Source: three-view drawing plus pictorial views. Frame: mm from the lowest corner of the part. Round coordinates to 2 decimals unless told otherwise and drop trailing zeros. Loops run counter-clockwise (first coordinate to the right, second up) from the corner with the lowest first, then second, coordinate; pieces in that order, holes last. Notation, with made-up numbers: M -16.75,47 L 8.25,47 A22 ccw 8.25,81 Z; hole C 5.25,-24 d4. An arc over 180 degrees is marked long. Write each question's results on one line, items separated by ' | '.
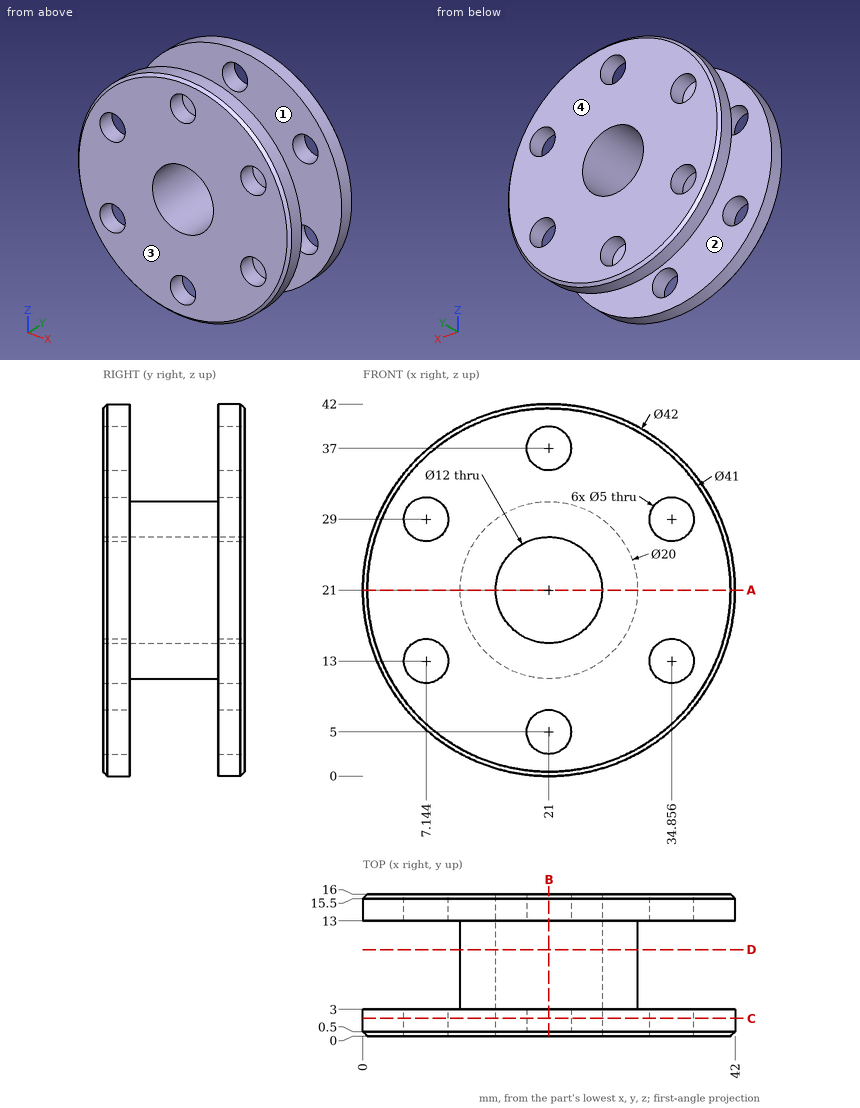
1. Pin query (flat end, axial travel): P1, Ø3, axis at x = 7.14, z = 13, coming from the -Y side; P2, Ø6, axis at x = 25.5, y = 11.5, coming from the +Z side; P3, Ø2, axis at x = 17, y = 7, coming from the +Z side; P4, Ø4, axis at x = 26, y = 12.5, coming from the -Z side (1 decimal). Return the tip coordinate at first contact, or that it passes through.
Answer key:
P1: passes through | P2: stops at z = 41.91 | P3: stops at z = 30.54 | P4: stops at z = 0.2
2. Ray query, probe 1 along Z at (x, y) = (21, 15.1); probe 2 along Z at (x, y) = (22, 15) (1 decimal); probe 3 along Y at (x, z) = (32, 18). Return the intervals inside material, ascending.
Answer key:
probe 1: z = 0 to 2.5, 7.5 to 15, 27 to 34.5, 39.5 to 42 | probe 2: z = 0 to 2.7, 7.3 to 15.1, 26.9 to 34.7, 39.3 to 42 | probe 3: y = 0 to 3, 13 to 16
3. Section D-D (y = 9.75). Output: boundary loops of the cut face in (x, z).
Answer key:
outline: C 21,21 d20; hole C 21,21 d12
4. Draft query along Y for the marked faces 1, 2, 3 and 4. Return one class per face: pulls with the +Y half, pulls with the -Y half, needs draft (parallel to the pull), parting line crosses it, or undercut.
Answer key:
face 1: undercut | face 2: undercut | face 3: pulls with the -Y half | face 4: pulls with the +Y half
5. Section A-A (z = 21). Output: boundary loops of the cut face in (x, y).
Answer key:
outline: M 0,0.5 L 0.5,0 L 15,0 L 15,16 L 0.5,16 L 0,15.5 L 0,13 L 11,13 L 11,3 L 0,3 Z; M 27,0 L 41.5,0 L 42,0.5 L 42,3 L 31,3 L 31,13 L 42,13 L 42,15.5 L 41.5,16 L 27,16 Z
6. Section C-C (y = 2). Output: boundary loops of the cut face in (x, z) (1 decimal), then the cut area to 3 significant figures.
Answer key:
outline: C 21,21 d42; hole C 7.1,13 d5; hole C 7.1,29 d5; hole C 21,21 d12; hole C 21,5 d5; hole C 21,37 d5; hole C 34.9,13 d5; hole C 34.9,29 d5 | area: 1,150 mm²
7. Section B-B (x = 21). Count the separate pieces of the cut face and the enclosed holes in it.
Answer key:
separate pieces: 6 | enclosed holes: 0
